Check sheet for the drawn part. Datum: minimum x, y, z corner. Units: mm. Coordinates: 2 decimals unless noted, no trailing zeros. Loops run counter-clockwise (first coordinate to the right, second up) from the corner with the lowest first, then second, coordinate; pieces in that order, holes last. Notation, with made-up numbers: M 25,39 L 76,39 A21 ccw 76,69 Z; hole C -37.75,8 d7. An arc over 180 degrees is marked long. Use CSV: the item, a comma, the result in double quotes. Start each with the question number.
(1) Scan lines: line 1 (X direction, y = 36, z = 0.25); line 2 (X direction, y = 49, z = 1.9). Record each from-to range of solid material in increasing order.
(2) Section check A-A on z = 0.35. Record the cut outline in (x, y).
(3) Go/stop test with a flat-tipped pin: pin 1 Ø8 at (x, y) = (81.5, 35) entering from -Z. Record where the tip stops, or that it passes through.
(4) Section check B-B on y = 38. Record the cut outline in (x, z).
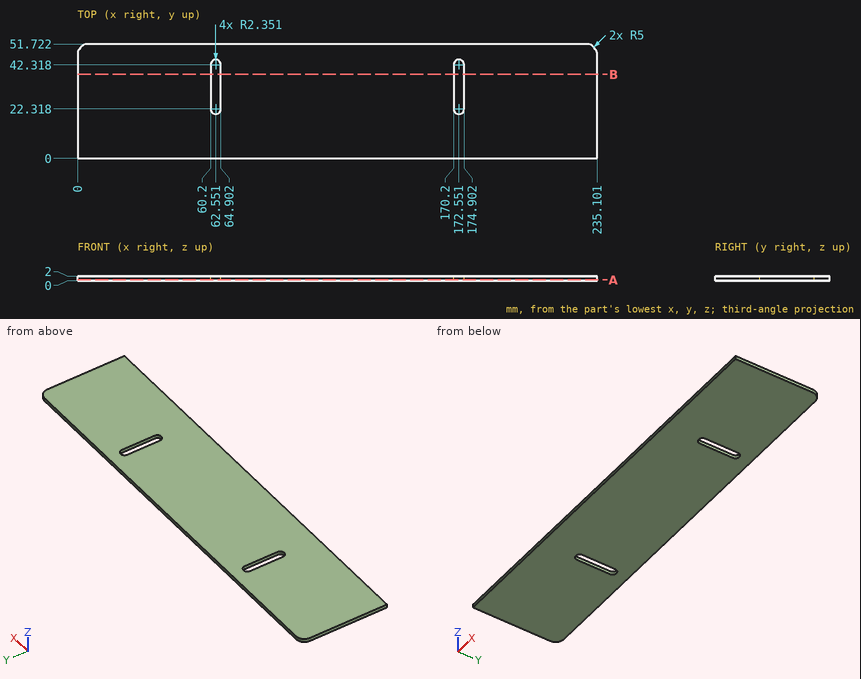
Outcome:
1,line 1,"x = 0 to 60.2, 64.9 to 170.2, 174.9 to 235.1"
1,line 2,"x = 0.55 to 234.55"
2,outline,"M 0,0 L 235.1,0 L 235.1,46.72 A5 ccw 230.1,51.72 L 5,51.72 A5 ccw 0,46.72 Z; hole M 60.2,22.32 A2.35 ccw 64.9,22.32 L 64.9,42.32 A2.35 ccw 60.2,42.32 Z; hole M 170.2,22.32 A2.35 ccw 174.9,22.32 L 174.9,42.32 A2.35 ccw 170.2,42.32 Z"
3,pin 1,"stops at z = 0"
4,outline,"M 0,0 L 60.2,0 L 60.2,2 L 0,2 Z; M 64.9,0 L 170.2,0 L 170.2,2 L 64.9,2 Z; M 174.9,0 L 235.1,0 L 235.1,2 L 174.9,2 Z"
